Verification items for the finished model (mm, model axes). A direction names the side the tool comes from. Round coordinates to 2 decimals unless told otherwise and drop trailing zeros. Order: outer loops, then holes, each group sorted by start corner. A loop starts at its lowest first (then second) coordinate and runs counter-clockwise, first axis right, second up. Notation, with made-up numbers: (82.25, -12) -> (130.25, -12) arc R23 ccw to (130.25, 15) -> close; hole circle Ø10 at (34, 25). An arc over 180 degrees is marked (long way). Put each result on its own line as item: value.
```python
from build123d import *

# Parameters (mm, degrees)
REVOLUTION004_ANGLE     = 180
SKETCH055_W             = 14
SKETCH055_H             = 6
PAD024_DEPTH            = 10
SKETCH054_R             = 1.7
POCKET003_DEPTH         = 39.401
POCKET004_DEPTH         = 29.401
BODY012_PLACEMENT_ANGLE = 180


with BuildPart() as part:
    # Sketch053 → Revolution004 (revolve, symmetric)
    with BuildSketch(Plane.YZ) as revolution004_sk:
        with BuildLine():
            Line((33.4, 0), (33.4, 6.5))
            Line((33.4, 6.5), (29.9, 6.5))
            ThreePointArc((28.4, 8), (28.83934, 6.93934), (29.9, 6.5))
            Line((28.4, 8), (28.4, 11))
            ThreePointArc((29.9, 12.5), (28.83934, 12.06066), (28.4, 11))
            Line((29.9, 12.5), (33.4, 12.5))
            ThreePointArc((39.4, 6.5), (37.642641, 10.742641), (33.4, 12.5))
            Line((39.4, 6.5), (39.4, 0))
            Line((39.4, 0), (39.4, -6.5))
            ThreePointArc((33.4, -12.5), (37.642641, -10.742641), (39.4, -6.5))
            Line((33.4, -12.5), (29.9, -12.5))
            ThreePointArc((28.4, -11), (28.83934, -12.06066), (29.9, -12.5))
            Line((28.4, -11), (28.4, -8))
            ThreePointArc((29.9, -6.5), (28.83934, -6.93934), (28.4, -8))
            Line((29.9, -6.5), (33.4, -6.5))
            Line((33.4, -6.5), (33.4, 0))
        make_face()
    revolve(axis=Axis((0, 0, 0), (0, 0, 1)), revolution_arc=REVOLUTION004_ANGLE / 2)
    revolve(revolution004_sk.sketch, axis=Axis((0, 0, 0), (0, 0, -1)), revolution_arc=REVOLUTION004_ANGLE / 2)

    # Sketch055 (on Face18 of Revolution004) → Pad024 (new body)
    with BuildSketch(Plane(origin=(0, 0, 0), x_dir=(0, 0, -1), z_dir=(0, -1, 0))):
        with Locations((0, 39.4)):
            Rectangle(SKETCH055_W, SKETCH055_H)
        with Locations((0, -39.4)):
            Rectangle(SKETCH055_W, SKETCH055_H)
    extrude(amount=-PAD024_DEPTH)

    # Sketch054 (on Face18 of Revolution004) → Pocket003 (cut, through all)
    with BuildSketch(Plane(origin=(0, 0, 0), x_dir=(0, 0, -1), z_dir=(0, -1, 0))):
        with Locations((4, 39.4)):
            Circle(SKETCH054_R)
        with Locations((-4, 39.4)):
            Circle(SKETCH054_R)
        with Locations((-4, -39.4)):
            Circle(SKETCH054_R)
        with Locations((4, -39.4)):
            Circle(SKETCH054_R)
    extrude(amount=-POCKET003_DEPTH, mode=Mode.SUBTRACT)

    # Sketch056 (on Face22 of Pocket003) → Pocket004 (cut, through all)
    with BuildSketch(Plane.ZX.offset(10)):
        with BuildLine():
            Line((-4, 43.4), (4.000001, 43.4))
            ThreePointArc((4.000001, 35.4), (8, 39.4), (4.000001, 43.4))
            Line((-4, 35.4), (4.000001, 35.4))
            ThreePointArc((-4, 43.4), (-8, 39.4), (-4, 35.4))
        make_face()
        with BuildLine():
            Line((-4, -35.4), (4, -35.4))
            ThreePointArc((4, -43.4), (8, -39.4), (4, -35.4))
            Line((-4, -43.4), (4, -43.4))
            ThreePointArc((-4, -35.4), (-8, -39.4), (-4, -43.4))
        make_face()
    extrude(amount=POCKET004_DEPTH, mode=Mode.SUBTRACT)


with BuildPart() as part_1:
    # Body012 placement: moved
    add(part.part.moved(Location((0, 0, -0.5))).rotate(Axis((0, 0, -0.5), (1, 0, 0)), BODY012_PLACEMENT_ANGLE))


solid = part_1.part
```
Item 1: Tool access check on faces 4 (the face through (35.4, -14, 0)), 5 (the face through (-35.85, -12.79, -6.34)), 6 (the face through (-0.645, -39.395, -0.409)), 7 (the face through (-41, -5, 6.5)), 8 (the face through (-2, -30, -7)). Record the directions out of +Z, -Z, +X, -X, +Y, -Y that give a thin tool (end or side, any length) a straight path to the whole face; none if there is none.
Geometry check:
face 4: +X, -Y
face 5: -X, -Y
face 6: +Z, -Z, -Y
face 7: +Z, -X, -Y
face 8: +Y
Item 2: Sectioned sample at B-B, the plane x = 0. Record the boundary of the cut face in (y, z).
Geometry check:
outline: (-39.4, -7) arc R6 ccw to (-33.4, -13) -> (-29.9, -13) arc R1.5 ccw to (-28.4, -11.5) -> (-28.4, -8.5) arc R1.5 ccw to (-29.9, -7) -> (-33.4, -7) -> (-33.4, 6) -> (-29.9, 6) arc R1.5 ccw to (-28.4, 7.5) -> (-28.4, 10.5) arc R1.5 ccw to (-29.9, 12) -> (-33.4, 12) arc R6 ccw to (-39.4, 6) -> close
Item 3: Depth check by flat-ended pin: pin 1 Ø10 at (y, z) = (-18, -5) entering from +X; pin 2 Ø6 at (y, z) = (-13.5, 8.5) entering from +X; pin 3 Ø5.5 at (x, z) = (-38.5, 2) entering from -Y; pin 4 Ø2 at (x, z) = (-39.4, -4.5) entering from -Y. Enter the tip coordinate at first touch or a pass-through.
Geometry check:
pin 1: x = 36.89
pin 2: x = 37.77
pin 3: y = -10
pin 4: through
Item 4: Sectioned sample at A-A, the plane y = -4.5. Give the number of separate pieces and of enclosed holes in the cut face, then the cut area to 3 significant figures.
Geometry check:
separate pieces: 2
enclosed holes: 4
area: 444 mm2
Item 5: Release check for a two-part mould opening along Z. For faces 1 (the face through (35, 0, -1)), 2 (the face through (41.086, -4.93, -4.721)), 3 (the face through (3, -30, -13)) record: pulls with the +Z half, pulls with the -Z half, needs draft (parallel to the pull), parting line crosses it, or undercut.
Geometry check:
face 1: needs draft
face 2: undercut
face 3: pulls with the -Z half
Item 6: Sectioned sample at C-C, the plane z = -1. Record the boundary of the cut face in (x, y), then the cut area to 3 significant figures.
Geometry check:
outline: (-42.4, -10) -> (-35.4, -10) -> (-35.4, -17.3) arc R39.4 ccw to (35.4, -17.3) -> (35.4, -10) -> (42.4, -10) -> (42.4, 0) -> (33.4, 0) arc R33.4 cw to (-33.4, 0) -> (-42.4, 0) -> close
area: 733 mm2
Item 7: Material ranges on line 1 along Z through (x, y) = (-23.5, -22.5); line 2 along X through (y, z) = (-3, -4) (3 decimals); line 3 along X through (y, z) = (-5.5, -4.5), recorded low to high.
Geometry check:
line 1: -13 to -7, 6 to 12
line 2: -42.4 to -41.025, -37.775 to -33.265, 33.265 to 37.775, 41.025 to 42.4
line 3: -42.4 to -41.1, -37.7 to -32.94, 32.94 to 37.7, 41.1 to 42.4
